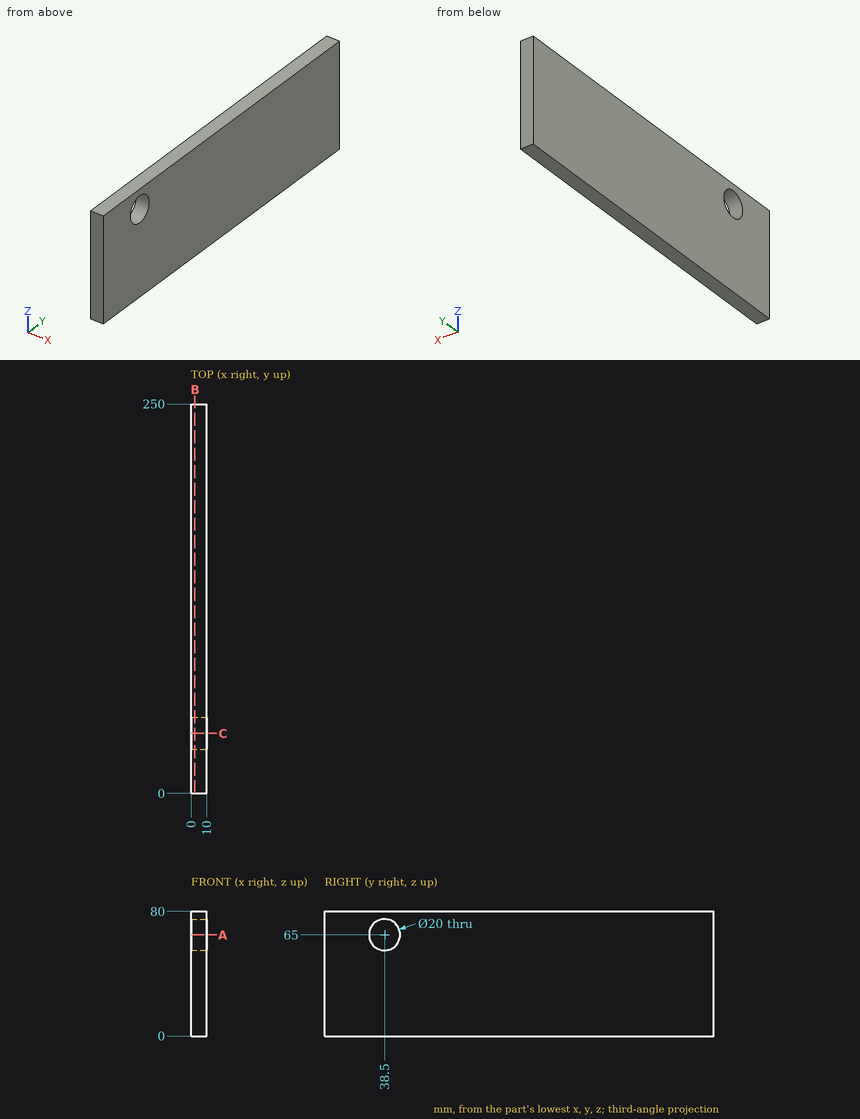
Can you work these out from the drawing? Everything is in mm from the part's minimum corner. Coordinates: 2 decimals unless noted, no trailing zeros. Loops run counter-clockwise (first coordinate to the right, second up) from the corner with the lowest first, then second, coordinate; pieces in that order, holes last. Notation, with made-up numbers: (-22, 31) -> (1, 31) arc R24 ccw to (1, 60) -> close; hole circle Ø11 at (43.5, 22.25). An arc over 180 degrees is marked (long way). Return JSON: item names as keys, results as strings.
1) If we section it at C-C, the plane y = 38.5: Write out the boundary of the cut face in (x, z), then the cut area to 3 significant figures.
Results below:
{"outline": "(0, 0) -> (10, 0) -> (10, 55) -> (0, 55) -> close; (0, 75) -> (10, 75) -> (10, 80) -> (0, 80) -> close", "area": "600 mm²"}
2) If we section it at A-A, the plane z = 65: Write out the boundary of the cut face in (x, y), then the cut area to 3 significant figures.
Results below:
{"outline": "(0, 0) -> (10, 0) -> (10, 28.5) -> (0, 28.5) -> close; (0, 48.5) -> (10, 48.5) -> (10, 250) -> (0, 250) -> close", "area": "2,300 mm²"}
3) I need wall thicknesses on line 1 (Z direction, x = 3.25, y = 38.5); line 2 (Y direction, x = 3.5, z = 72.5); line 3 (Y direction, x = 1.5, z = 70). Which ranges of each line are inside material? Lowest first, please. Write a range as from..to.
Results below:
{"line 1": "0..55, 75..80", "line 2": "0..31.89, 45.11..250", "line 3": "0..29.84, 47.16..250"}
4) If we section it at B-B, the plane x = 2.5: Write out the boundary of the cut face in (y, z), then the cut area to 3 significant figures.
Results below:
{"outline": "(0, 0) -> (250, 0) -> (250, 80) -> (0, 80) -> close; hole circle Ø20 at (38.5, 65)", "area": "19,700 mm²"}
